Input: dimensioned drawing with shaded views. Units: mm. Origin: part minimum x, y, z. A direction names the side the tool comes from. Round coordinates to 2 decimals unless told otherwise and drop trailing zeros. Loops run counter-clockwise (first coordinate to the right, second up) from the corner with the lowest first, then second, coordinate; pieces in that order, holes last.
Item 1: Section query A-A on x = 2.25. Return loops of the section in (y, z).
Item 2: First-contact query: P1, Ø1.8, axis at x = 7.5, z = 2.5, coming from the +Y side; P2, Ø5, axis at y = 20, z = 8, coming from the -X side; P3, Ø1.4, axis at x = 2, z = 8, coming from the -Y side; P4, Ø3.5, axis at y = 7, z = 3.5, coming from the -X side (3 decimals). Flat tips, straight axial feed; report the tip coordinate or a pass-through.
Item 3: Section query B-B on y = 20. Return loops of the section in (x, z) (1 decimal).
Item 4: Access query for the marked faces 1, 2 and 3. Directions: +Z, -Z, +X, -X, +Y, -Y. A direction counts if a zero-diameter tool reaches every point of the face in a straight line with its end or side. Return the directions, or none.
Item 5: Section query C-C on z = 1. Return loops of the section in (x, y) (1 decimal), then the cut area to 3 significant figures.
Item 6: Section query D-D on x = 26.5. Return loops of the section in (y, z).
Item 7: Ray query, L1, parallel to Z at x = 2.25, y = 16.4; L2, parallel to X at y = 12.5, z = 11 (1 decimal); L3, parallel to Y at x = 26, z = 3.25. Return the intervals inside material, ascending.
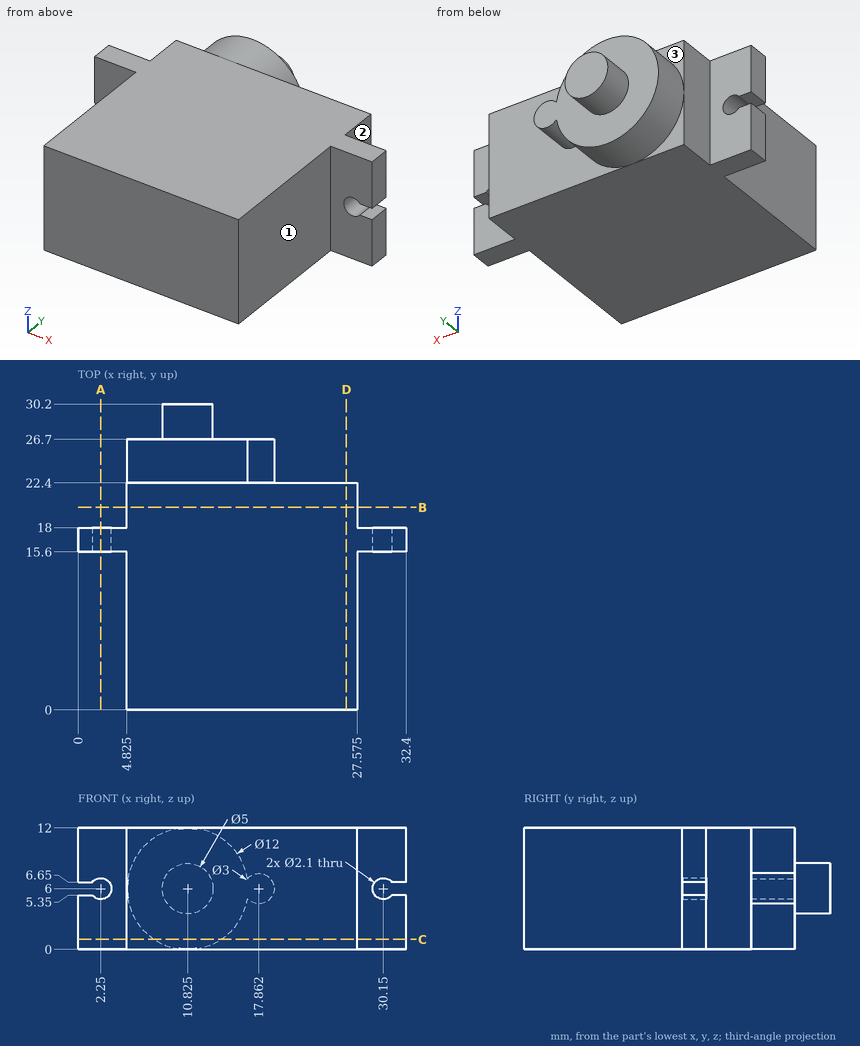
Data:
1. outline: (15.6, 0) - (18, 0) - (18, 4.95) - (15.6, 4.95) - close; (15.6, 7.05) - (18, 7.05) - (18, 12) - (15.6, 12) - close
2. P1: stops at y = 26.7
2. P2: stops at x = 0
2. P3: stops at y = 15.6
2. P4: stops at x = 4.825
3. outline: (4.8, 0) - (27.6, 0) - (27.6, 12) - (4.8, 12) - close
4. face 1: +Z, -Z, +X, -Y
4. face 2: +Z, -Z, +X, +Y
4. face 3: +Z, -X, +Y
5. outline: (0, 15.6) - (4.8, 15.6) - (4.8, 0) - (27.6, 0) - (27.6, 15.6) - (32.4, 15.6) - (32.4, 18) - (27.6, 18) - (27.6, 22.4) - (14.1, 22.4) - (14.1, 26.7) - (7.5, 26.7) - (7.5, 22.4) - (4.8, 22.4) - (4.8, 18) - (0, 18) - close
5. area: 561 mm2
6. outline: (0, 0) - (22.4, 0) - (22.4, 12) - (0, 12) - close
7. L1: z = 0 to 4.95, 7.05 to 12
7. L2: x = 4.8 to 27.6
7. L3: y = 0 to 22.4
